Model file for the job. Use its own axes, mm. Round coordinates to 2 decimals unless told otherwise and drop trailing zeros. Order: outer loops, then holes, each group sorted by start corner. A loop starts at its lowest first (then second) coordinate and runs counter-clockwise, first axis right, second up. Notation, with made-up numbers: (4, 39) - (42, 39) arc R34 ccw to (42, 74) - close; hole circle Ø3 at (67, 73). An arc over 180 degrees is marked (long way). Put each result on its own line as item: value. Start each with the question number.
Item 1: Probe probe 1 along Y at (x, z) = (87.9, 0.5); probe 2 along Y at (x, z) = (0, 2.45); probe 3 along X at (y, z) = (64.9, 2.5). List the from-to ranges inside material, lowest first.
Item 2: Saw through at A-A on x = 42.5. List the corners of the cut face in (y, z), plus the area to 3 significant figures.
Item 3: Pin check, flat tips, straight feed: pin 1 Ø3 at (x, y) = (87.9, 0) entering from +Z; pin 2 Ø2 at (x, y) = (88, 64) entering from -Z; pin 3 Ø10.5 at (x, y) = (87.9, 0) entering from -Z. Stop position of each tip, or through.
Item 4: Saw through at C-C on y = 40.5. List the corners of the cut face in (x, z).
Item 5: Saw through at B-B on y = 76.15. List the corners of the cut face in (x, z), plus the area to 3 significant figures.
Item 6: Saw through at D-D on x = 54. List the corners of the cut face in (y, z).
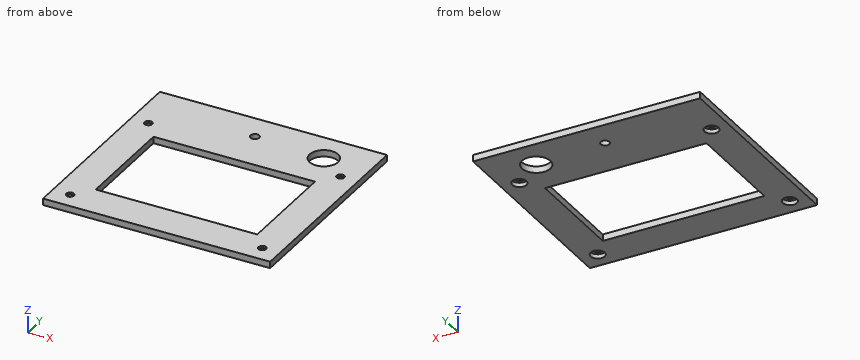
```python
from build123d import *

# Parameters (mm, degrees)
SKETCH1_R           = 1.75
SKETCH1_R_2         = 6.5
SKETCH1_R_3         = 2
SKETCH1_W           = 77.9
SKETCH1_H           = 47.9
BOSS_EXTRUDE1_DEPTH = 3
SKETCH2_W           = 2
SKETCH2_H           = 47.9
BOSS_EXTRUDE2_DEPTH = 3
SKETCH4_W           = 15
SKETCH4_H           = 92.738679811
BOSS_EXTRUDE4_DEPTH = 3
SKETCH5_W           = 15
SKETCH5_H           = 92.013865939
BOSS_EXTRUDE5_DEPTH = 3
SKETCH7_W           = 103.9
SKETCH7_H           = 15
BOSS_EXTRUDE6_DEPTH = 3
SKETCH9_R           = 3.25
CUT_EXTRUDE1_DEPTH  = 2
SKETCH10_W          = 103.9
SKETCH10_H          = 15
BOSS_EXTRUDE8_DEPTH = 3
SKETCH12_R          = 3.75
SKETCH12_R_2        = 1.75
BOSS_EXTRUDE9_DEPTH = 8
SKETCH13_W          = 3
SKETCH13_H          = 23
CUT_EXTRUDE2_DEPTH  = 8
SKETCH14_W          = 281.555590783
SKETCH14_H          = 173.736843818
CUT_EXTRUDE3_DEPTH  = 12


with BuildPart() as part:
    # Sketch1 → Boss-Extrude1 (new body)
    with BuildSketch(Plane.XY):
        Polygon((-5, -5), (-5, 69.9), (-5, 85.9), (92.9, 85.9), (92.9, 69.9), (92.9, -5), align=None)
        with Locations((0, 64.9)):
            Circle(SKETCH1_R, mode=Mode.SUBTRACT)
        with Locations((87.9, 64.9)):
            Circle(SKETCH1_R, mode=Mode.SUBTRACT)
        with Locations((87.9, 0)):
            Circle(SKETCH1_R, mode=Mode.SUBTRACT)
        Circle(SKETCH1_R, mode=Mode.SUBTRACT)
        with Locations((75, 74.4)):
            Circle(SKETCH1_R_2, mode=Mode.SUBTRACT)
        with Locations((42.5, 76.15)):
            Circle(SKETCH1_R_3, mode=Mode.SUBTRACT)
        with Locations((43.95, 32.45)):
            Rectangle(SKETCH1_W, SKETCH1_H, mode=Mode.SUBTRACT)
    extrude(amount=BOSS_EXTRUDE1_DEPTH)

    # Sketch2 → Boss-Extrude2 (add)
    with BuildSketch(Plane.XY.offset(3)):
        with Locations((81.9, 32.45)):
            Rectangle(SKETCH2_W, SKETCH2_H)
        with Locations((6, 32.45)):
            Rectangle(SKETCH2_W, SKETCH2_H)
    extrude(amount=-BOSS_EXTRUDE2_DEPTH)

    # Sketch4 → Boss-Extrude4 (add)
    with BuildSketch(Plane(origin=(92.9, 0, 0), x_dir=(0, 0, -1), z_dir=(1, 0, 0))):
        with Locations((-7.5, 41.369339906)):
            Rectangle(SKETCH4_W, SKETCH4_H)
    extrude(amount=BOSS_EXTRUDE4_DEPTH)

    # Sketch5 → Boss-Extrude5 (add)
    with BuildSketch(Plane.ZY.offset(5)):
        with Locations((7.5, 41.006932969)):
            Rectangle(SKETCH5_W, SKETCH5_H)
    extrude(amount=BOSS_EXTRUDE5_DEPTH)

    # Sketch7 → Boss-Extrude6 (add)
    with BuildSketch(Plane(origin=(0, -5, 0), x_dir=(-1, 0, 0), z_dir=(0, -1, 0))):
        with Locations((-43.95, -7.5)):
            Rectangle(SKETCH7_W, SKETCH7_H)
    extrude(amount=BOSS_EXTRUDE6_DEPTH)

    # Sketch9 → Cut-Extrude1 (cut)
    with BuildSketch(Plane(origin=(0, 0, 0), x_dir=(-1, 0, 0), z_dir=(0, 0, -1))):
        Circle(SKETCH9_R)
        with Locations((-87.9, 0)):
            Circle(SKETCH9_R)
        with Locations((-87.9, 64.9)):
            Circle(SKETCH9_R)
        with Locations((0, 64.9)):
            Circle(SKETCH9_R)
    extrude(amount=-CUT_EXTRUDE1_DEPTH, mode=Mode.SUBTRACT)

    # Sketch10 → Boss-Extrude8 (add)
    with BuildSketch(Plane(origin=(0, 85.9, 0), x_dir=(1, 0, 0), z_dir=(0, 1, 0))):
        with Locations((43.95, -7.5)):
            Rectangle(SKETCH10_W, SKETCH10_H)
    extrude(amount=BOSS_EXTRUDE8_DEPTH)

    # Sketch12 → Boss-Extrude9 (add)
    with BuildSketch(Plane.XY.offset(3)):
        with Locations((0, 64.9)):
            Circle(SKETCH12_R)
        with Locations((0, 64.9)):
            Circle(SKETCH12_R_2, mode=Mode.SUBTRACT)
        Circle(SKETCH12_R)
        Circle(SKETCH12_R_2, mode=Mode.SUBTRACT)
        with Locations((87.9, 64.9)):
            Circle(SKETCH12_R)
        with Locations((87.9, 64.9)):
            Circle(SKETCH12_R_2, mode=Mode.SUBTRACT)
        with Locations((87.9, 0)):
            Circle(SKETCH12_R)
        with Locations((87.9, 0)):
            Circle(SKETCH12_R_2, mode=Mode.SUBTRACT)
    extrude(amount=BOSS_EXTRUDE9_DEPTH)

    # Sketch13 → Cut-Extrude2 (cut)
    with BuildSketch(Plane(origin=(95.9, 0, 0), x_dir=(0, 0, -1), z_dir=(1, 0, 0))):
        with Locations((-13.5, 53.54685285)):
            Rectangle(SKETCH13_W, SKETCH13_H)
    extrude(amount=-CUT_EXTRUDE2_DEPTH, mode=Mode.SUBTRACT)

    # Sketch14 → Cut-Extrude3 (cut)
    with BuildSketch(Plane.XY.offset(15)):
        with Locations((95.022411609, 36.684941712)):
            Rectangle(SKETCH14_W, SKETCH14_H)
    extrude(amount=-CUT_EXTRUDE3_DEPTH, mode=Mode.SUBTRACT)


solid = part.part
```
Results found:
1. probe 1: y = -8 to -3.25, 3.25 to 61.65, 68.15 to 88.9
1. probe 2: y = -8 to -1.75, 1.75 to 63.15, 66.65 to 88.9
1. probe 3: x = -8 to -1.75, 1.75 to 86.15, 89.65 to 95.9
2. outline: (-8, 0) - (8.5, 0) - (8.5, 3) - (-8, 3) - close; (56.4, 0) - (74.15, 0) - (74.15, 3) - (56.4, 3) - close; (78.15, 0) - (88.9, 0) - (88.9, 3) - (78.15, 3) - close
2. area: 135 mm²
3. pin 1: passes through
3. pin 2: stops at z = 2
3. pin 3: stops at z = 0
4. outline: (-8, 0) - (7, 0) - (7, 3) - (-8, 3) - close; (80.9, 0) - (95.9, 0) - (95.9, 3) - (80.9, 3) - close
5. outline: (-8, 0) - (40.5, 0) - (40.5, 3) - (-8, 3) - close; (44.5, 0) - (68.74, 0) - (68.74, 3) - (44.5, 3) - close; (81.26, 0) - (95.9, 0) - (95.9, 3) - (81.26, 3) - close
5. area: 262 mm²
6. outline: (-8, 0) - (8.5, 0) - (8.5, 3) - (-8, 3) - close; (56.4, 0) - (88.9, 0) - (88.9, 3) - (56.4, 3) - close
